Geometry: final body of the model. Coordinates: model frame, mm. Face numbers are marked on the shaded views. A direction names the side the tool comes from. Round coordinates to 2 decimals unless told otherwise and drop trailing zeros. Order: outer loops, then holes, each group sorted by start corner. A loop starts at its lowest first (then second) coordinate and runs counter-clockwise, first axis right, second up. Notation, with made-up numbers: (63.5, 33.5) -> (99.5, 33.5) arc R14 cw to (99.5, 41.5) -> close; hole circle Ø2 at (74, 8.25). An arc over 180 degrees is marked (long way). Put each result on its own line as item: value.
Autodesk Fusion 360 part; units mm, degrees
sketch "Sketch1" plane through (0, 0, 0) normal (0, 1, 0) x (1, 0, 0)
  line L0 (0, 0) -> (19, 0)
  line L1 (19, 0) -> (19, 90)
  line L2 (19, 90) -> (0, 90)
  line L3 (0, 90) -> (0, 0)
  dimension "d1" = 19
  dimension "d2" = 90
extrude "Extrude1" add sketch "Sketch1" along normal blind 50
sketch "Sketch2" plane through (19, 0, 0) normal (1, 0, 0) x (0, 0, -1)
  line L0 (0, 0) -> (90, 0)
  line L1 (90, 0) -> (90, 50)
  line L2 (90, 50) -> (0, 50)
  line L3 (0, 50) -> (0, 0)
  circle A0 centre (14.125, 14.125) radius 11.125
  line L4 (28.25, 45) -> (85, 45)
  line L5 (85, 45) -> (85, 15)
  line L6 (85, 15) -> (28.25, 15)
  line L7 (28.25, 15) -> (28.25, 45)
  circle A1 centre (14.125, 14.125) radius 14.125
  dimension "d5" = 22.25
  dimension "d7" = 5
  dimension "d8" = 15
  dimension "d9" = 5
  dimension "d10" = 30
  dimension "d24" = 3
extrude "Extrude2" cut sketch "Sketch2" against normal up to surface (19 mm away) contours L0 L3 A1 | A0 | L4 L5 L6 L7
fillet "Fillet1" radius 30 1 edges at (9.5, 50, 0)
sketch "Sketch3" plane through (0, 0, -90) normal (0, 0, -1) x (-1, 0, 0)
  line L0 (-19, 0) -> (0, 0)
  line L1 (0, 0) -> (0, 50)
  line L2 (0, 50) -> (-19, 50)
  line L3 (-19, 50) -> (-19, 0)
  circle A0 centre (-9.5, 32.5) radius 6.5
  line L4 (-9.5, 50) -> (-9.5, 0) construction
  line L5 (-19, 32.5) -> (0, 32.5) construction
  dimension "d17" = 13
  dimension "d29" = 17.5
extrude "Extrude3" cut sketch "Sketch3" against normal up to surface (5 mm away) contours A0
fillet "Fillet2" radius 15 1 edges at (9.5, 15, -85)
fillet "Fillet2" radius 5 1 edges at (9.5, 45, -85)
fillet "Fillet3" radius 15 2 edges at (9.5, 45, -28.25) (9.5, 15, -28.25)
chamfer "Chamfer1" distance 11 distance2 70 1 edges at (9.5, 0, -90) measured on face at (9.6619, 8.6727, -90)
equation "d6 = d5"
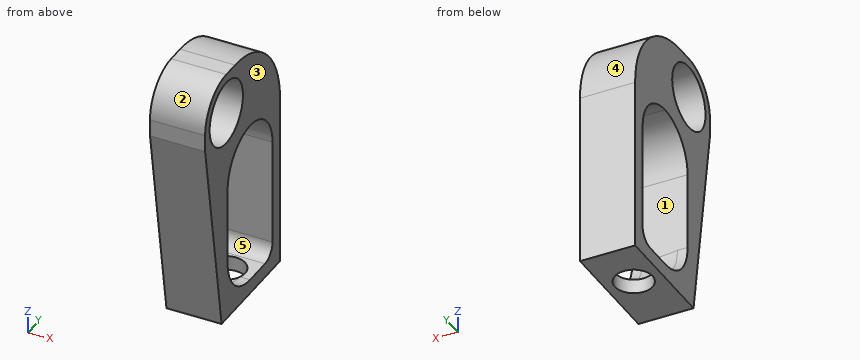
1. Cut plane B-B on z = -21.5. Return loops of the section in (x, y), and give its area (3 significant figures).
Ans:
outline: (0, 0.24) -> (19, 0.24) -> (19, 5.8) -> (0, 5.8) -> close; (0, 22.45) -> (19, 22.45) -> (19, 48.77) -> (0, 48.77) -> close
area: 606 mm²
2. Draft query along Z for the marked faces 3, 4 and 5. Return one class per face: +Z half, -Z half, draft (parallel to the pull), parting line (faces both ways), or undercut.
Ans:
face 3: draft
face 4: +Z half
face 5: undercut
3. Material intervals for probe 1 along X at (y, z) = (32, -87); probe 2 along Z at (x, y) = (7.25, 20.5); probe 3 along Z at (x, y) = (13, 21.5), sorted ascending.
Ans:
probe 1: 0 to 3.02, 15.98 to 19
probe 2: -90 to -82.05, -31.64 to -23.24, -5.01 to 0
probe 3: -90 to -82.66, -30.89 to -22.45, -5.8 to -0.04
4. Contact query for flat-ended pins moving along their axis: P1, Ø20, axis at y = 14.125, z = -14.125, coming from the +X side; P2, Ø10, axis at x = 3.5, y = 39.5, coming from the +Z side; P3, Ø4, axis at x = 11.5, z = -10.5, coming from the +Y side; P4, Ø5, axis at x = 5, z = -72.5, coming from the -Y side. Output: stop coordinate, or through.
Ans:
P1: through
P2: z = -3.74
P3: y = 44.37
P4: y = 7.86
5. Cut plane C-C on z = -53.5. Return loops of the section in (x, y), and give its area (3 significant figures).
Ans:
outline: (0, 5.26) -> (19, 5.26) -> (19, 15) -> (0, 15) -> close; (0, 45) -> (19, 45) -> (19, 50) -> (0, 50) -> close
area: 280 mm²
6. Set-up query: the marked faces 1 and 2. Return all of +Z, -Z, +X, -X, +Y, -Y with unobstructed straight access to the full face (end or side cutting, diameter ignored); none if empty.
Ans:
face 1: +X, -X
face 2: +Z, +X, -X, -Y
7. Cut plane A-A on y = 32.5. Return loops of the section in (x, z).
Ans:
outline: (0, -90) -> (3, -90) -> (3, -85) -> (0, -85) -> close; (0, -28.46) -> (19, -28.46) -> (19, -2.73) -> (0, -2.73) -> close; (16, -90) -> (19, -90) -> (19, -85) -> (16, -85) -> close
